from build123d import *

# Parameters (mm, degrees)
SKETCH2_R          = 5
CUT_EXTRUDE1_DEPTH = 7
SKETCH3_R          = 2
CUT_EXTRUDE2_DEPTH = 7
FILLET1_R          = 1


with BuildPart() as part:
    # Sketch1 → Revolve1 (revolve)
    with BuildSketch(Plane(origin=(0, 0, 0), x_dir=(1, 0, 0), z_dir=(0, 1, 0))):
        Polygon((0, 0), (0, 13), (7.5, 13), (11, 0), align=None)
    revolve(axis=Axis((0, 0, 0), (0, 0, -1)))

    # Sketch2 → Cut-Extrude1 (cut)
    with BuildSketch(Plane(origin=(0, 0, -13), x_dir=(-1, 0, 0), z_dir=(0, 0, -1))):
        Circle(SKETCH2_R)
    extrude(amount=-CUT_EXTRUDE1_DEPTH, mode=Mode.SUBTRACT)

    # Sketch3 → Cut-Extrude2 (cut, through all)
    with BuildSketch(Plane(origin=(0, 0, -6), x_dir=(-1, 0, 0), z_dir=(0, 0, -1))):
        Circle(SKETCH3_R)
    extrude(amount=-CUT_EXTRUDE2_DEPTH, mode=Mode.SUBTRACT)

    # Fillet1
    fillet1_edges = [part.edges().sort_by_distance(p)[0] for p in [
        (5, 0, -13),
        (-11, 0, 0),
        (-7.5, 0, -13),
    ]]
    fillet(fillet1_edges, radius=FILLET1_R)


solid = part.part
Verification items for the finished model (mm, model axes). A direction names the side the tool comes from. Give positions to 0.01 mm unless a question says otherwise; leave off trailing zeros. Order: outer loops, then holes, each group sorted by start corner. A loop starts at its lowest first (then second) coordinate and runs counter-clockwise, first axis right, second up. Notation, with made-up numbers: M 41.5,37.25 L 99.5,37.25 A27 cw 99.5,54.25 Z; hole C 16.5,-30 d2. An arc over 180 degrees is marked long. Answer as a JSON object with one key per item and string values. Group by question number.
1) Cross-section at C-C (z = -5.5). Enter the section's corners in (x, y), then the cut area to 3 significant figures.
2) Cross-section at D-D (z = -9.5). Enter the section's corners in (x, y).
3) Depth check by flat-ended pin: pin 1 Ø6 at (y, z) = (6.5, -10) entering from -X; pin 2 Ø5 at (x, y) = (-2.5, -1.5) entering from -Z; pin 3 Ø1 at (x, z) = (-3, -5) entering from -Y. Enter the tip coordinate at first touch or a pass-through.
4) Cross-section at A-A (x = 0). Enter the section's corners in (y, z).
5) Access from +Z, -Z, +X, -X, +Y, -Y to the whole of each face (thin tool, end or side, straight path). Record for faces 4 (the face through (0.1, -2.2, -6)), 5 (the face through (0, -2, -3)).
6) Mould release check, pull along Y, two halves, no side actions. Record for faces 1 (the face through (8.148, -2.566, -9.127)), 2 (the face through (1.08, -4.88, -9.04)), 3 (the face through (-2.3, -0.1, 0)): released by +Y, released by -Y, zero draft, split by the parting line, or undercut.
7) Scan lines: line 1 along Y through (x, z) = (0, -9.5); line 2 along Z through (x, y) = (1.5, 1.5); line 3 along Y through (x, z) = (1.75, -4). Record each from-to range of solid material in increasing order. Write a range as [from, to].
Result sheet:
{
 "1": {"outline": "C 0,0 d19.04; hole C 0,0 d4", "area": "272 mm2"},
 "2": {"outline": "C 0,0 d16.88; hole C 0,0 d10"},
 "3": {"pin 1": "stops at x = -7.79", "pin 2": "stops at z = -12.81", "pin 3": "stops at y = -9.38"},
 "4": {"outline": "M -10.66,-1.26 L -7.7,-12.26 A1 ccw -6.73,-13 L -6,-13 A1 ccw -5,-12 L -5,-6 L -2,-6 L -2,0 L -9.7,0 A1 ccw Z; M 2,-6 L 5,-6 L 5,-12 A1 ccw 6,-13 L 6.73,-13 A1 ccw 7.7,-12.26 L 10.66,-1.26 A1 ccw 9.7,0 L 2,0 Z"},
 "5": {"face 4": "-Z", "face 5": "+Z, -Z"},
 "6": {"face 1": "split by the parting line", "face 2": "undercut", "face 3": "zero draft"},
 "7": {"line 1": "y = [-8.44, -5], [5, 8.44]", "line 2": "z = [-6, 0]", "line 3": "y = [-9.77, -0.97], [0.97, 9.77]"}
}
